```python
from build123d import *

# Parameters (mm, degrees)
BOSS_EXTRUDE1_DEPTH = 3.175
CUT_EXTRUDE1_DEPTH  = 401.46617672


with BuildPart() as part:
    # Sketch3 → Boss-Extrude1 (new body)
    with BuildSketch(Plane(origin=(0, -90.186626134, -561.928406554), x_dir=(1, 0, 0), z_dir=(0, 0.15846690258874493, 0.9873642898059101))):
        with BuildLine():
            Line((374.396, 137.827848871), (374.396, 141.63269915))
            add(Edge.make_bspline(
                [(374.396, 141.63269915), (365.378247241, 140.351869422), (356.378821901, 138.957098969), (338.401992935, 136.030650092), (329.424670358, 134.498314058), (313.750786532, 131.748061478), (307.051747759, 130.548427396), (300.355738535, 129.33221679)],
                knots=[0, 0, 0, 0, 0.25, 0.25, 0.5, 0.5, 0.68681431, 0.68681431, 0.68681431, 0.68681431], degree=3))
            Line((300.355738535, 129.33221679), (301.717495498, 121.834882733))
            add(Edge.make_bspline(
                [(371.221, 133.4767647), (366.485652047, 132.785360934), (355.611621495, 131.127793525), (338.582430164, 128.339546997), (320.149202977, 125.153673819), (307.858393043, 122.950267206), (301.717495498, 121.834882733)],
                knots=[0.039503599, 0.039503599, 0.039503599, 0.039503599, 0.171703578, 0.343407155, 0.515110733, 0.68681431, 0.68681431, 0.68681431, 0.68681431], degree=3))
            Line((371.221, 133.4767647), (371.221, 137.827848871))
            Line((371.221, 137.827848871), (374.396, 137.827848871))
        make_face()
    extrude(amount=BOSS_EXTRUDE1_DEPTH)

    # Sketch4 → Cut-Extrude1 (cut, through all)
    with BuildSketch(Plane(origin=(0, -90.186626134, -561.928406554), x_dir=(-1, 0, 0), z_dir=(-9.1104866082071e-14, -0.158466902588134, -0.9873642898060083))):
        Polygon((-323.025447556, 125.638791395), (-323.025447556, 123.807923692), (-319.861053503, 123.734597093), (-319.861053503, 125.083150774), (-319.773665288, 129.384296303), (-322.948038155, 129.448791395), align=None)
    extrude(amount=-CUT_EXTRUDE1_DEPTH, mode=Mode.SUBTRACT)


solid = part.part
```
Can you work these out from the model? Positions are in its coordinate system, mm. A direction names the side the tool comes from. Coordinates: 2 decimals unless noted, no trailing zeros.
1. Thinking about a two-plate mould opening in X: for faces 3 (the face through (336.858, 40.019, -582.826)), 4 (the face through (374.396, 48, -583)), which applies, +X half, -X half, draft (parallel to the pull), parting line (faces both ways), or undercut?
2. I'm going to push flat-ended pins straight in: pin 1 (1.5 mm diameter, centred on y = 36.5, z = -582, fed in from -X); pin 2 (0.6 mm diameter, centred on y = 34, z = -580.5, fed in from -X); pin 3 (2 mm diameter, centred on x = 314, z = -579.5, fed in from +Y). Where does each tip first touch, or does it pass through?
3. I need wall thicknesses on line 1 (Z direction, x = 347.5, y = 45.25); line 2 (Z direction, x = 364, y = 47.25); line 3 (Y direction, x = 304, z = -580). Which ranges of each line are inside material? Lowest first, please.
4. For faces 1 (the face through (336.86, 40.52, -579.69)), 2 (the face through (372.79, 46.15, -582.22)), which set-ups out of +Z, -Z, +X, -X, +Y, -Y let a thin tool reach every point of the face, with its end or its side?
Entries:
1. face 3: draft
1. face 4: +X half
2. pin 1: stops at x = 300.41
2. pin 2: stops at x = 300.99
2. pin 3: stops at y = 40.61
3. line 1: z = -583.67 to -580.45
3. line 2: z = -583.99 to -580.77
3. line 3: y = 30.73 to 38.57
4. face 1: +Z, +X, -X, +Y
4. face 2: +Z, +X, -Y
